For this review, take the finished solid that the model builds, in its own axes (mm). Face numbers are marked on the shaded views. A direction names the side the tool comes from. Coordinates: 2 decimals unless noted, no trailing zeros. Order: outer loops, then holes, each group sorted by start corner. A loop starts at its lowest first (then second) coordinate and runs counter-clockwise, first axis right, second up. Notation, with made-up numbers: M 19,24.5 L 28,24.5 A23 ccw 28,56.5 Z; hole C -40,-19 d5. An arc over 180 degrees is marked long. Use CSV: the item, a comma, the result in double quotes.
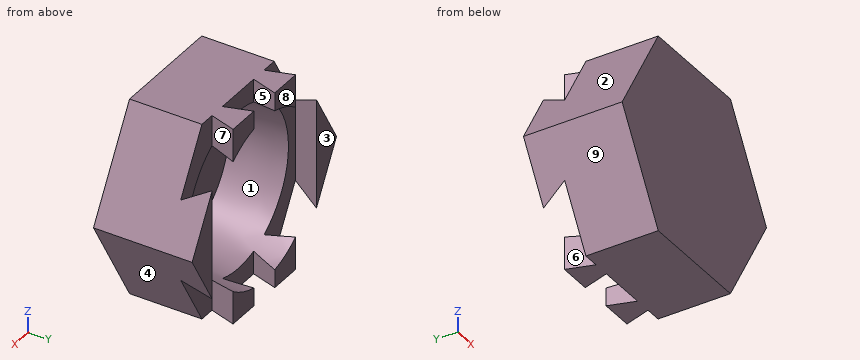
```python
from build123d import *

# Parameters (mm, degrees)
EXTRUDE_1_DEPTH               = 30
CUT_EXTRUDE_1_DEPTH           = 55.772255751
PATTERN_LINEAR_1_COUNT        = 2
PATTERN_LINEAR_1_PITCH        = 20
PATTERN_LINEAR_2_COPY_1_DEPTH = 55.772255751
PATTERN_LINEAR_2_COPY_2_DEPTH = 55.772255751


with BuildPart() as part:
    # 草圖1 → 填料-伸長1 (new body)
    with BuildSketch(Plane(origin=(0, 0, 0), x_dir=(1, 0, 0), z_dir=(0, 1, 0))):
        Polygon((17.320508076, -30), (34.641016151, 0), (17.320508076, 30), (-17.320508076, 30), (-34.641016151, 0), (-17.320508076, -30), align=None)
    extrude(amount=EXTRUDE_1_DEPTH)

    # 草圖2 → 除料-旋轉1 (revolve, cut)
    with BuildSketch(Plane.XY):
        Polygon((0, 30), (25, 30), (22.5, 5), (0, 5), align=None)
    revolve(axis=Axis((0, 5, 0), (0, 1, 0)), mode=Mode.SUBTRACT)

    # 草圖3 → 除料-伸長1 (cut, symmetric)
    with BuildSketch(Plane.XY):
        Polygon((-5, 30), (-7.5, 22), (7.5, 22), (5, 30), align=None)
    cut_extrude_1 = extrude(amount=CUT_EXTRUDE_1_DEPTH, both=True, mode=Mode.SUBTRACT)

    # 直線複製排列1: 除料-伸長1 ×2
    with Locations(*[(-i * PATTERN_LINEAR_1_PITCH, 0, 0) for i in range(1, PATTERN_LINEAR_1_COUNT)]):
        add(cut_extrude_1, mode=Mode.SUBTRACT)

    # 直線複製排列2 copy 1 sketch → 直線複製排列2 copy 1 (cut, symmetric)
    with BuildSketch(Plane.XY):
        Polygon((-5, 30), (-7.5, 22), (7.5, 22), (5, 30), align=None)
    extrude(amount=PATTERN_LINEAR_2_COPY_1_DEPTH, both=True, mode=Mode.SUBTRACT)

    # 直線複製排列2 copy 2 sketch → 直線複製排列2 copy 2 (cut, symmetric)
    with BuildSketch(Plane(origin=(20, 0, 0), x_dir=(1, 0, 0), z_dir=(0, 0, 1))):
        Polygon((-5, 30), (-7.5, 22), (7.5, 22), (5, 30), align=None)
    extrude(amount=PATTERN_LINEAR_2_COPY_2_DEPTH, both=True, mode=Mode.SUBTRACT)


solid = part.part
```
Item 1: Draft analysis for pull direction Z (two halves, no side actions). For the marked faces 1, 2, 3 and 4, state which applies: released by +Z, released by -Z, zero draft, split by the parting line, or undercut.
Solutions:
face 1,"undercut"
face 2,"released by +Z"
face 3,"zero draft"
face 4,"released by -Z"
Item 2: Add section C-C on y = 19. State the section outline as (x, z) points, and give its area (3 significant figures).
Solutions:
outline,"M -34.64,0 L -17.32,-30 L 17.32,-30 L 34.64,0 L 17.32,30 L -17.32,30 Z; hole C 0,0 d47.8"
area,"1,320 mm^2"
Item 3: To check wall thickness, follow line 1 along Y through (x, z) = (-11.5, -4); line 2 along Z through (x, y) = (11.5, 25.5); line 3 along Z through (x, y) = (-14, 12). State the ranges of each line that lie inside material, in increasing order. Write a range as [from, to].
Solutions:
line 1,"[0, 5]"
line 2,"[-30, -21.69], [21.69, 30]"
line 3,"[-30, -18.5], [18.5, 30]"
Item 4: Clearance check with flat-ended pins moving along their axes: pin 1 Ø1.5 at (y, z) = (15, 8) entering from +X; pin 2 Ø1.5 at (y, z) = (3, -15) entering from +X; pin 3 Ø2 at (x, z) = (1, -25.5) entering from +Y. State where each tip first meets the part, or that it passes through.
Solutions:
pin 1,"x = 30.46"
pin 2,"x = 26.41"
pin 3,"y = 22"
Item 5: For the marked faces 5, 6, 7, 8 and 9, list the 3-axis set-ups (+Z, -Z, +X, -X, +Y, -Y) from which the entire face can be reached by the end or side of a thin tool; tool diameter is ignored.
Solutions:
face 5,"+Z, -Z"
face 6,"+Z, -Z, -X"
face 7,"+Z, -Z, +X"
face 8,"+Z, -Z, +X, -X, +Y"
face 9,"-Z, -X, +Y, -Y"
Item 6: Add section B-B on y = 26. State the section outline as (x, z) points.
Solutions:
outline,"M -34.64,0 L -26.25,-14.53 L -26.25,14.53 Z; M -13.75,-30 L -6.25,-30 L -6.25,-23.79 A24.6 cw -13.75,-20.4 Z; M -13.75,20.4 A24.6 cw -6.25,23.79 L -6.25,30 L -13.75,30 Z; M 6.25,-30 L 13.75,-30 L 13.75,-20.4 A24.6 cw 6.25,-23.79 Z; M 6.25,23.79 A24.6 cw 13.75,20.4 L 13.75,30 L 6.25,30 Z; M 26.25,-14.53 L 34.64,0 L 26.25,14.53 Z"
Item 7: Add section A-A on x = 0. State the section outline as (y, z) points.
Solutions:
outline,"M 0,-30 L 22,-30 L 22,-24.2 L 5,-22.5 L 5,22.5 L 22,24.2 L 22,30 L 0,30 Z"
